For this review, take the finished solid that the model builds, in its own axes (mm). Face numbers are marked on the shaded views. A direction names the side the tool comes from. Give positions to 0.01 mm unless a question says otherwise; leave off trailing zeros. Write each loop counter-clockwise with the first axis right and the second up, starting at its lowest first coordinate (ties: lowest second). Pieces come first, ordered by that corner, then holes.
1) Wall thickness on line 1 along X through (y, z) = (6.25, -7.62); line 2 along X through (y, z) = (3.5, -46.99); line 3 along Z through (x, y) = (16, 0.5): over which ranges is each line inside the solid? List them lowest first.
2) We need section B-B on z = 8. Give the boundary of the cut face in (x, y).
3) We need section C-C on y = -17.5. Give the boundary of the cut face in (x, z).
4) We need section A-A on y = 4.5. Give the boundary of the cut face in (x, z).
5) For P1, Ø7.5, axis at x = 18.49, z = -46.99, coming from the +Y side; P2, Ø0.8, axis at x = 3.5, y = -9, coming from the +Z side; P3, Ø10, axis at x = 3, z = 10.5, coming from the +Y side; P4, Ø3, axis at x = 21, y = -15, coming from the +Z side, all flat-tipped, find the tip position at first contact; note any pin that passes through.
6) We need section D-D on z = 27. Give the boundary of the cut face in (x, y).
7) Machinability: for the marked faces 1 and 2, which of the approach directions +Z, -Z, +X, -X, +Y, -Y give a long, thin tool a straight path to every point of the face, cutting with its end or side? Answer none if there is none.
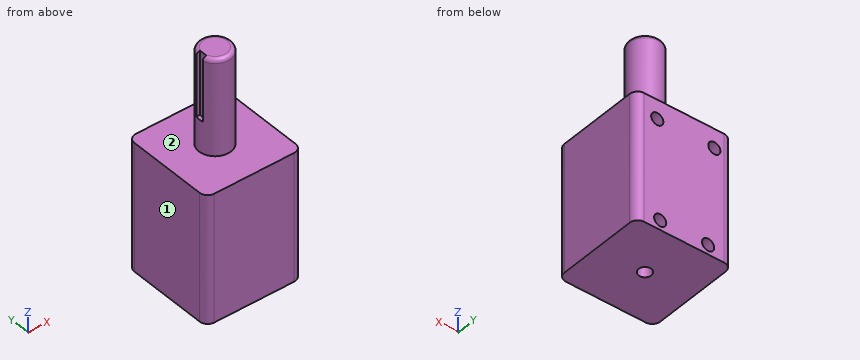
Autodesk Inventor part; units mm, degrees
ref_plane "YZ Plane" through (0, 0, 0) normal (1, 0, 0) x (0, 1, 0)
ref_plane "XZ Plane" through (0, 0, 0) normal (0, 1, 0) x (-1, 0, 0)
ref_plane "XY Plane" through (0, 0, 0) normal (0, 0, 1) x (1, 0, 0)
sketch "Sketch1" plane through (0, 0, 0) normal (0, 0, 1) x (1, 0, 0)
  line L0 (-10.0849, -28.7582) -> (28.0151, -28.7582)
  line L1 (28.0151, -28.7582) -> (28.0151, 9.3418)
  line L2 (28.0151, 9.3418) -> (-10.0849, 9.3418)
  line L3 (-10.0849, 9.3418) -> (-10.0849, -28.7582)
  circle A0 centre (8.9651, -9.7082) radius 6.35
  point P0 (0, 0)
  point P1 (8.9651, 9.3418)
  point P2 (-10.0849, -9.7082)
  dimension "d0" = 38.1
  dimension "d1" = 38.1
  dimension "d4" = 12.7
extrude "Extrusion1" add sketch "Sketch1" against normal blind 50.8 contours L3 L2 L1 L0 | A0
extrude "Extrusion2" add sketch "Sketch1" along normal blind 38.1 contours A0
fillet "Fillet1" radius 1.5875 1 edges at (2.6151, -9.7082, 38.1)
fillet "Fillet2" radius 3.175 4 edges at (28.0151, 9.3418, -25.4) (-10.0849, 9.3418, -25.4) (28.0151, -28.7582, -25.4) (-10.0849, -28.7582, -25.4)
sketch "Sketch2" plane through (8.9651, -9.7082, 38.1) normal (0, 0, 1) x (1, 0, 0)
  circle A0 centre (0, 0) radius 4.7625
  line L0 (-4.7625, -1.5875) -> (-4.7625, 1.5875)
  line L1 (-4.7625, 1.5875) -> (-7.9375, 1.5875)
  line L2 (-7.9375, 1.5875) -> (-7.9375, -1.5875)
  line L3 (-7.9375, -1.5875) -> (-4.7625, -1.5875)
  point P0 (-8.9651, 9.7082)
  dimension "d13" = 3.175
  dimension "d14" = 1.5875
  dimension "d15" = 3.175
extrude "Extrusion3" cut sketch "Sketch2" against normal blind 25.4 contours L0 L3 L2 L1
sketch "Sketch3" plane through (-6.9099, 9.3418, 0) normal (0, 1, 0) x (1, 0, 0)
  line L0 (31.75, 0) -> (0, 0)
  line L1 (31.75, 50.8) -> (0, 50.8)
  line L2 (-3.175, 50.8) -> (-3.175, 0)
  point P0 (6.9099, 0)
  point P1 (26.5665, 7.62)
  point P2 (25.4, 46.99)
  point P3 (6.35, 46.99)
  point P4 (3.8887, 7.62)
  point P5 (34.925, 50.8)
  dimension "d18" = 7.62
  dimension "d19" = 7.62
  dimension "d20" = 3.81
  dimension "d21" = 3.81
  dimension "d22" = 9.525
  dimension "d23" = 9.525
hole "Hole1" at (19.6566, 9.3418, -7.62) at (18.4901, 9.3418, -46.99) at (-0.5599, 9.3418, -46.99) at (-3.0212, 9.3418, -7.62) direction (0, -1, 0) diameter 4.826 depth 7.62 tip angle 118
thread "Thread1"
thread "Thread2"
thread "Thread3"
thread "Thread4"
sketch "Sketch4" plane through (0, 0, -50.8) normal (0, 0, -1) x (-1, 0, 0)
  point P0 (0, 0)
  point P1 (-8.9651, -9.7082)
hole "Hole2" at (8.9651, -9.7082, -50.8) direction (0, 0, 1) diameter 5.08 depth 7.62 tip angle 118
properties part number "p60 gearbox proxy"
Results list:
1. line 1: x = -10.08 to -5.43, -0.61 to 17.24, 22.07 to 28.01
1. line 2: x = -10.08 to -2.97, 1.85 to 16.08, 20.9 to 28.02
1. line 3: z = -50.8 to 0
2. outline: circle Ø12.7 at (8.97, -9.71)
3. outline: (-10.08, -50.8) - (28.02, -50.8) - (28.02, 0) - (-10.08, 0) - close
4. outline: (-10.08, -50.8) - (28.02, -50.8) - (28.02, 0) - (-10.08, 0) - close; hole circle Ø4.83 at (-3.02, -7.62); hole circle Ø4.83 at (-0.56, -46.99); hole circle Ø4.83 at (18.49, -46.99); hole circle Ø4.83 at (19.66, -7.62)
5. P1: stops at y = 9.34
5. P2: stops at z = 12.7
5. P3: stops at y = -3.43
5. P4: stops at z = 0
6. outline: (2.82, -11.3) arc R6.35 ccw (long way) to (2.82, -8.12) - (4.2, -8.12) - (4.2, -11.3) - close
7. face 1: +Z, -Z, -X, +Y, -Y
7. face 2: +Z
